Autodesk Inventor part; units mm, degrees
ref_plane "YZ Plane" through (0, 0, 0) normal (1, 0, 0) x (0, 1, 0)
ref_plane "XZ Plane" through (0, 0, 0) normal (0, 1, 0) x (-1, 0, 0)
ref_plane "XY Plane" through (0, 0, 0) normal (0, 0, 1) x (1, 0, 0)
sketch "Boceto1" plane through (0, 0, 0) normal (0, 0, 1) x (1, 0, 0)
  line L0 (0, 0) -> (135, 0)
  line L1 (0, 0) -> (0, 40)
  line L2 (0, 40) -> (25, 40)
  line L3 (25, 40) -> (25, 25)
  line L4 (25, 25) -> (20, 25)
  line L5 (20, 25) -> (20, 20)
  line L6 (20, 20) -> (140, 20) construction
  line L7 (135, 0) -> (135, 15) construction
  line L8 (135, 0) -> (135, 15)
  line L9 (135, 15) -> (140, 15)
  line L10 (140, 15) -> (140, 20)
  line L11 (20, 20) -> (80, 20) construction
  line L12 (80, 20) -> (80, 22.5) construction
  line L13 (80, 22.5) -> (80, 17.5) construction
  line L14 (20, 20) -> (80, 17.5)
  line L15 (80, 17.5) -> (80, 22.5)
  line L16 (80, 22.5) -> (140, 20)
  dimension "d0" = 135
  dimension "d1" = 40
  dimension "d2" = 25
  dimension "d3" = 15
  dimension "d4" = 5
  dimension "d5" = 5
  dimension "d6" = 120
  dimension "d7" = 15
  dimension "d9" = 5
  dimension "d10" = 60
  dimension "d11" = 2.5
  dimension "d12" = 5
extrude "Extrusión1" add sketch "Boceto1" along normal blind 40
sketch "Boceto2" plane through (0, 0, 0) normal (0, -1, 0) x (1, 0, 0)
  line L0 (0, 0) -> (79.9, 0)
  line L1 (25, 0) -> (0, 0)
  line L2 (79.9, 0) -> (79.9, 20)
  line L3 (0, 0) -> (135, 0)
  line L4 (79.9, 0) -> (99.9, 0) construction
  line L5 (79.9, 20) -> (49.9, 20)
  line L6 (80, 0) -> (80, 40)
  line L7 (79.9, 20) -> (109.9, 20) construction
  line L8 (79.9, 20) -> (109.9, 20)
  line L9 (79.9, 20) -> (109.9, 20) construction
  line L10 (47.4, 17.5) -> (52.4, 17.5)
  line L11 (52.4, 17.5) -> (52.4, 22.5)
  line L12 (52.4, 22.5) -> (47.4, 22.5)
  line L13 (47.4, 22.5) -> (47.4, 17.5)
  line L14 (47.4, 17.5) -> (52.4, 22.5) construction
  line L15 (52.4, 17.5) -> (47.4, 22.5) construction
  line L16 (107.4, 17.5) -> (112.4, 17.5)
  line L17 (112.4, 17.5) -> (112.4, 22.5)
  line L18 (112.4, 22.5) -> (107.4, 22.5)
  line L19 (107.4, 22.5) -> (107.4, 17.5)
  line L20 (107.4, 17.5) -> (112.4, 22.5) construction
  line L21 (112.4, 17.5) -> (107.4, 22.5) construction
  dimension "d15" = 79.9
  dimension "d16" = 20
  dimension "d17" = 90
  dimension "d18" = 30
  dimension "d19" = 180
  dimension "d20" = 30
  dimension "d21" = 0
  dimension "d22" = 5
  dimension "d23" = 5
  dimension "d24" = 5
  dimension "d25" = 5
extrude "Extrusión2" cut sketch "Boceto2" against normal blind 40 contours L11 L10 L13 L12 | L19 L18 L17 L16
equation "\"d3\" = Largo_rebaje - Correccion_rebaje"
equation "\"d4\" = Espesor_corte"
equation "\"d5\" = Espesor_corte"
equation "\"d9\" = Espesor_corte"
equation "\"d11\" = Espesor_detalle"
equation "\"d12\" = Espesor_corte"
equation "\"d15\" = Largo_segundo_boceto"
equation "\"d22\" = Espesor_corte"
equation "\"d23\" = Espesor_corte"
equation "\"d24\" = Espesor_corte"
equation "\"d25\" = Espesor_corte"
equation "\"Largo_rebaje\" = 20"
equation "\"Correccion_rebaje\" = 5"
equation "\"Espesor_corte\" = 5"
equation "\"Espesor_detalle\" = 2.5"
equation "\"Largo_segundo_boceto\" = 79.9"
properties part number "Hembra_parametrizada"
The model under review builds one solid part; all positions refer to its coordinate system, in mm. A direction names the side the tool comes from. Round coordinates to 2 decimals unless told otherwise and drop trailing zeros. Loops run counter-clockwise (first coordinate to the right, second up) from the corner with the lowest first, then second, coordinate; pieces in that order, holes last. Notation, with made-up numbers: (-12.5, -6.75) -> (9.5, -6.75) arc R19 ccw to (9.5, 6.25) -> close; hole circle Ø4 at (-20, 73.5). An arc over 180 degrees is marked (long way). Write item = value, one per line. Start each with the question number.
Item 1: Take a section at A-A on y = 4. Give the boundary of the cut face in (x, z).
Item 2: Insertion check: pin 1 (2.5 mm diameter, centred on y = 22.5, z = 18.5, fed in from +X); pin 2 (10 mm diameter, centred on x = 86.5, y = 28, fed in from +Z); pin 3 (12 mm diameter, centred on y = 32, z = 15, fed in from +X); pin 4 (5.5 mm diameter, centred on y = 10, z = 20.5, fed in from +X). Each pin has a flat end and moves straight along its axis. Give the tip position at first contact, or say it passes through.
Item 3: Mouldability with a two-part tool opening along Z and no side actions: class faces 1 (the flat face through (69, 16, 0)), 2 (the flat face through (50, 9, 17.5)), 3 (the flat face through (47.4, 9, 20)), 4 (the flat face through (135, 7, 20)) as released by +Z, released by -Z, zero draft, split by the parting line, or undercut.
Item 4: Take a section at D-D on y = 35. Give the boundary of the cut face in (x, z).
Item 5: For faces 5 (the flat face through (80, 20, 20)), 6 (the flat face through (137, 15, 20)), 7 (the flat face through (25, 33, 20)), 8 (the flat face through (107.4, 11, 20)), 9 (the flat face through (20, 23, 20)), list the 3-axis set-ups (+Z, -Z, +X, -X, +Y, -Y) from which the entire face can be reached by the end or side of a thin tool; tool diameter is ignored.
Item 6: To check wall thickness, follow L1, parallel to X at y = 30, z = 3; L2, parallel to X at y = 12, z = 7; L3, parallel to Y at x = 79.5, z = 11. State the ranges of each line that lie inside material, in increasing order.
Item 7: Take a section at C-C on x = 21.5. Give the boundary of the cut face in (y, z).
Item 8: Take a section at B-B on z = 31. Give the boundary of the cut face in (x, y).
Result:
q1.outline = (0, 0) -> (135, 0) -> (135, 40) -> (0, 40) -> close; hole (47.4, 17.5) -> (52.4, 17.5) -> (52.4, 22.5) -> (47.4, 22.5) -> close; hole (107.4, 17.5) -> (112.4, 17.5) -> (112.4, 22.5) -> (107.4, 22.5) -> close
q2.pin_1 = 107.4
q2.pin_2 = through
q2.pin_3 = 25
q2.pin_4 = 135
q3.face_1 = released by -Z
q3.face_2 = undercut
q3.face_3 = undercut
q3.face_4 = zero draft
q4.outline = (0, 0) -> (25, 0) -> (25, 40) -> (0, 40) -> close
q5.face_5 = +Z, -Z, +Y
q5.face_6 = +Z, -Z, +X, -Y
q5.face_7 = +Z, -Z, +X, +Y
q5.face_8 = +Y, -Y
q5.face_9 = +Z, -Z
q6.L1 = 0 to 25
q6.L2 = 0 to 135
q6.L3 = 0 to 17.52
q7.outline = (0, 0) -> (19.94, 0) -> (19.94, 40) -> (0, 40) -> close; (25, 0) -> (40, 0) -> (40, 40) -> (25, 40) -> close
q8.outline = (0, 0) -> (135, 0) -> (135, 15) -> (140, 15) -> (140, 20) -> (80, 22.5) -> (80, 17.5) -> (20, 20) -> (20, 25) -> (25, 25) -> (25, 40) -> (0, 40) -> close
